from build123d import *

# Parameters (mm, degrees)
CROQUIS1_R              = 4
CROQUIS1_R_2            = 1.6
CROQUIS1_R_3            = 6.1
CROQUIS1_R_4            = 8.1
SALIENTE_EXTRUIR1_DEPTH = 3


with BuildPart() as part:
    # Croquis1 → Saliente-Extruir1 (new body)
    with BuildSketch(Plane.XY):
        Polygon((-127, 22.5), (-105, 40), (105, 40), (127, 22.5), (127, -22.5), (105, -40), (-105, -40), (-127, -22.5), align=None)
        with Locations((0, 20)):
            Circle(CROQUIS1_R, mode=Mode.SUBTRACT)
        with Locations((112.98, 25.35)):
            Circle(CROQUIS1_R_2, mode=Mode.SUBTRACT)
        with Locations((120.25, 0)):
            Circle(CROQUIS1_R_2, mode=Mode.SUBTRACT)
        with Locations((112.98, -25.35)):
            Circle(CROQUIS1_R_2, mode=Mode.SUBTRACT)
        with Locations((77.5, -33.9)):
            Circle(CROQUIS1_R_2, mode=Mode.SUBTRACT)
        with Locations((28.5, -33.9)):
            Circle(CROQUIS1_R_2, mode=Mode.SUBTRACT)
        with Locations((-28.5, -33.9)):
            Circle(CROQUIS1_R_2, mode=Mode.SUBTRACT)
        with Locations((-77.5, -33.9)):
            Circle(CROQUIS1_R_2, mode=Mode.SUBTRACT)
        with Locations((-112.98, -25.35)):
            Circle(CROQUIS1_R_2, mode=Mode.SUBTRACT)
        with Locations((-120.25, 0)):
            Circle(CROQUIS1_R_2, mode=Mode.SUBTRACT)
        with Locations((-112.98, 25.35)):
            Circle(CROQUIS1_R_2, mode=Mode.SUBTRACT)
        with Locations((-77.5, 33.9)):
            Circle(CROQUIS1_R_2, mode=Mode.SUBTRACT)
        with Locations((-28.5, 33.9)):
            Circle(CROQUIS1_R_2, mode=Mode.SUBTRACT)
        with Locations((28.5, 33.9)):
            Circle(CROQUIS1_R_2, mode=Mode.SUBTRACT)
        with Locations((77.5, 33.9)):
            Circle(CROQUIS1_R_2, mode=Mode.SUBTRACT)
        with Locations((-82.5, 0)):
            Circle(CROQUIS1_R_3, mode=Mode.SUBTRACT)
        with Locations((82.5, 0)):
            Circle(CROQUIS1_R_3, mode=Mode.SUBTRACT)
        with Locations((0, 5.55)):
            Circle(CROQUIS1_R_4, mode=Mode.SUBTRACT)
        with Locations((0, -16.95)):
            Circle(CROQUIS1_R_4, mode=Mode.SUBTRACT)
        with Locations((-7.8, 13.1)):
            Circle(CROQUIS1_R_2, mode=Mode.SUBTRACT)
        with Locations((75.5, 15.5)):
            Circle(CROQUIS1_R_2, mode=Mode.SUBTRACT)
        with Locations((75.5, -15.5)):
            Circle(CROQUIS1_R_2, mode=Mode.SUBTRACT)
        with Locations((62.076606241, -7.75)):
            Circle(CROQUIS1_R_2, mode=Mode.SUBTRACT)
        with Locations((88.923393759, -7.75)):
            Circle(CROQUIS1_R_2, mode=Mode.SUBTRACT)
        with Locations((-89.5, 15.5)):
            Circle(CROQUIS1_R_2, mode=Mode.SUBTRACT)
        with Locations((-102.923393759, -7.75)):
            Circle(CROQUIS1_R_2, mode=Mode.SUBTRACT)
        with Locations((-76.076606241, -7.75)):
            Circle(CROQUIS1_R_2, mode=Mode.SUBTRACT)
        with Locations((-89.5, -15.5)):
            Circle(CROQUIS1_R_2, mode=Mode.SUBTRACT)
    extrude(amount=SALIENTE_EXTRUIR1_DEPTH)


solid = part.part
Read the model definition and answer for the solid it produces. Units are mm, in the model's axes. Round coordinates to 2 decimals unless told otherwise and drop trailing zeros. Loops run counter-clockwise (first coordinate to the right, second up) from the corner with the lowest first, then second, coordinate; pieces in that order, holes last.
Q1. Section B-B on x = 0 is taken. Write down the section's boundary in (y, z), and give its area (3 significant figures).
Q2. Each of these flat-tipped pins is pushed along its axis until it touches: pin 1 (4 mm diameter, centred on x = -28.5, y = -33.9, fed in from -Z); pin 2 (7 mm diameter, centred on x = 0, y = 20, fed in from -Z). Where does it stop, or does it pass through?
Q3. Consider probe 1 along Y at (x, z) = (75.5, 1.05); probe 2 along X at (y, z) = (-16.5, 2.3); probe 3 along Y at (x, z) = (113.5, 0.4). Determine where each line is inside the solid, lowest interval first.
Q4. Determine the mould class of faces 1 (the face through (-116.15, 31.13, 1.48)), 2 (the face through (-1.756, -2.357, 1.479)), 3 (the face through (88.135, -2.336, 1.479)), 4 (the face through (2, -8, 3)) for opening direction X: released by +X, released by -X, zero draft, split by the parting line, or undercut.
Q5. Section A-A on x = -82.5 is taken. Write down the section's boundary in (y, z), and give its area (3 significant figures).
Q6. Section C-C on z = 1.3 is taken. Give the number of separate pieces and of enclosed holes in the cut face, and give its area (3 significant figures).
Output:
1. outline: (-40, 0) - (-25.05, 0) - (-25.05, 3) - (-40, 3) - close; (-8.85, 0) - (-2.55, 0) - (-2.55, 3) - (-8.85, 3) - close; (13.65, 0) - (16, 0) - (16, 3) - (13.65, 3) - close; (24, 0) - (40, 0) - (40, 3) - (24, 3) - close
1. area: 119 mm2
2. pin 1: stops at z = 0
2. pin 2: passes through
3. probe 1: y = -40 to -17.1, -13.9 to 13.9, 17.1 to 40
3. probe 2: x = -127 to -90.75, -88.25 to -8.09, 8.09 to 74.25, 76.75 to 127
3. probe 3: y = -33.24 to -26.86, -23.84 to 23.84, 26.86 to 33.24
4. face 1: released by -X
4. face 2: undercut
4. face 3: undercut
4. face 4: zero draft
5. outline: (-40, 0) - (-6.1, 0) - (-6.1, 3) - (-40, 3) - close; (6.1, 0) - (40, 0) - (40, 3) - (6.1, 3) - close
5. area: 203 mm2
6. separate pieces: 1
6. enclosed holes: 28
6. area: 18,700 mm2
